Study the drawing (mm; zero at the part's minimum x, y, z) and answer. A direction names the side the tool comes from. Round coordinates to 2 decimals unless told otherwise and drop trailing zeros. Order: outer loops, then holes, each group sorted by start corner. A loop starts at its lowest first (then second) coordinate and runs counter-clockwise, first axis right, second up. Notation, with made-up numbers: (74, 13.5) -> (111, 13.5) arc R23 cw to (111, 24.5) -> close; hole circle Ø3 at (80, -10). An arc over 180 degrees is marked (long way). Use one line per item in the form item = value.
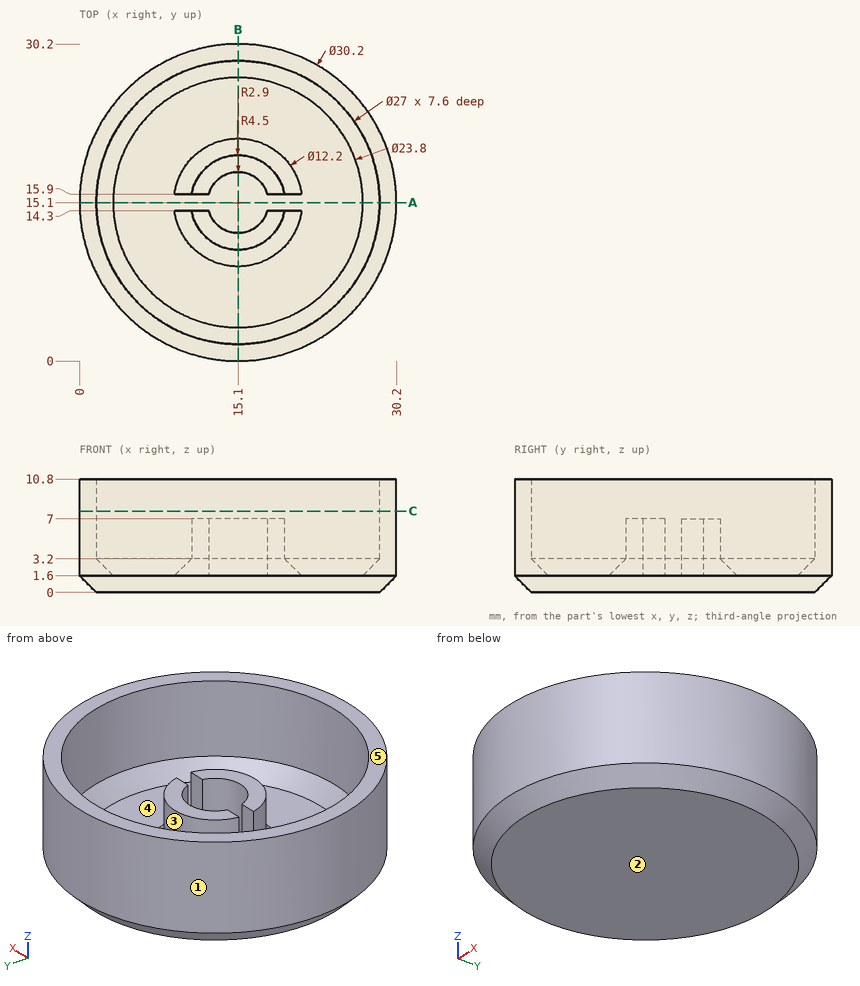
Item 1: The part is cut by section A-A, the plane y = 15.1. Give the vertices of the cut face in (x, z), and give its area (3 significant figures).
Findings:
outline = (0, 1.6) -> (1.6, 0) -> (28.6, 0) -> (30.2, 1.6) -> (30.2, 10.8) -> (28.6, 10.8) -> (28.6, 3.2) -> (27, 1.6) -> (3.2, 1.6) -> (1.6, 3.2) -> (1.6, 10.8) -> (0, 10.8) -> close
area = 77.8 mm^2
Item 2: Consider line 1 along Y through (x, z) = (15.1, 5); line 2 along Z through (x, y) = (26, 13.5); line 3 along Y through (x, z) = (15.1, 8.5). Determine where each line is inside the solid, lowest interval first.
Findings:
line_1 = 0 to 1.6, 10.6 to 12.2, 18 to 19.6, 28.6 to 30.2
line_2 = 0 to 1.6
line_3 = 0 to 1.6, 28.6 to 30.2
Item 3: The part is cut by section B-B, the plane x = 15.1. Give the vertices of the cut face in (y, z).
Findings:
outline = (0, 1.6) -> (1.6, 0) -> (28.6, 0) -> (30.2, 1.6) -> (30.2, 10.8) -> (28.6, 10.8) -> (28.6, 3.2) -> (27, 1.6) -> (21.2, 1.6) -> (19.6, 3.2) -> (19.6, 7) -> (18, 7) -> (18, 1.6) -> (12.2, 1.6) -> (12.2, 7) -> (10.6, 7) -> (10.6, 3.2) -> (9, 1.6) -> (3.2, 1.6) -> (1.6, 3.2) -> (1.6, 10.8) -> (0, 10.8) -> close
Item 4: Flat-ended cylindrical pins translate along their axes: P1, Ø1.5, axis at x = 8, z = 9, coming from the +Y side; P2, Ø2, axis at y = 10, z = 5, coming from the -X side; P3, Ø1.5, axis at y = 19.5, z = 2, coming from the +X side. Find the tip coordinate at first contact, or state that the pin passes through.
Findings:
P1 = 28.8
P2 = 0.57
P3 = 29.75
Item 5: The part is cut by section C-C, the plane z = 7.75. Give the vertices of the cut face in (x, y), and give its area (3 significant figures).
Findings:
outline = circle Ø30.2 at (15.1, 15.1); hole circle Ø27 at (15.1, 15.1)
area = 144 mm^2
Item 6: Determine the mould class of the marked faces 1, 2 and 3 for opening direction X: released by +X, released by -X, zero draft, split by the parting line, or undercut.
Findings:
face_1 = split by the parting line
face_2 = zero draft
face_3 = undercut
Item 7: For the marked faces 4 and 5, determine the directions among +Z, -Z, +X, -X, +Y, -Y from which every point of the face is accessible in a straight line to the end or side of a thin tool.
Findings:
face_4 = +Z
face_5 = +Z, +X, -X, +Y, -Y
